from build123d import *

# Parameters (mm, degrees)
SKETCH1_W           = 125
SKETCH1_H           = 100
BOSS_EXTRUDE1_DEPTH = 15
SKETCH2_R           = 50
SKETCH2_R_2         = 37.5
BOSS_EXTRUDE2_DEPTH = 25
SKETCH5_R           = 20
BOSS_EXTRUDE3_DEPTH = 25
SKETCH6_R           = 15
CUT_EXTRUDE2_DEPTH  = 15


with BuildPart() as part:
    # Sketch1 → Boss-Extrude1 (new body)
    with BuildSketch(Plane(origin=(0, 0, 0), x_dir=(1, 0, 0), z_dir=(0, 1, 0))):
        Rectangle(SKETCH1_W, SKETCH1_H)
    boss_extrude1 = extrude(amount=BOSS_EXTRUDE1_DEPTH)

    # Sketch2 → Boss-Extrude2 (add)
    with BuildSketch(Plane.XZ):
        Circle(SKETCH2_R)
        Circle(SKETCH2_R_2, mode=Mode.SUBTRACT)
    extrude(amount=BOSS_EXTRUDE2_DEPTH)

    # Sketch5 → Boss-Extrude3 (add)
    with BuildSketch(Plane(origin=(62.5, 0, 0), x_dir=(0, 0, -1), z_dir=(1, 0, 0))):
        with BuildLine():
            ThreePointArc((-50, 100), (0, 150), (50, 100))
            Line((50, 100), (50, 15))
            Line((50, 15), (-50, 15))
            Line((-50, 15), (-50, 100))
        make_face()
        with Locations((0, 100)):
            Circle(SKETCH5_R, mode=Mode.SUBTRACT)
    boss_extrude3 = extrude(amount=-BOSS_EXTRUDE3_DEPTH)

    # Mirror1: Boss-Extrude1, Boss-Extrude3 across plane
    add(boss_extrude1.mirror(Plane(origin=(0, 0, 0), x_dir=(0, 0, 1), z_dir=(1, 0, 0))))
    add(boss_extrude3.mirror(Plane(origin=(0, 0, 0), x_dir=(0, 0, 1), z_dir=(1, 0, 0))))

    # Sketch6 → Cut-Extrude2 (cut)
    with BuildSketch(Plane.XZ):
        Circle(SKETCH6_R)
    extrude(amount=-CUT_EXTRUDE2_DEPTH, mode=Mode.SUBTRACT)


solid = part.part
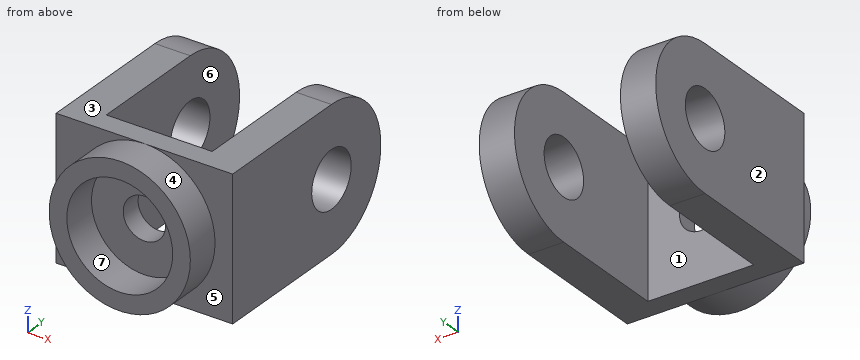
CAD build for the part. Positions are in the model's coordinates, mm. Face numbers are marked on the shaded views. A direction names the side the tool comes from. Round coordinates to 2 decimals unless told otherwise and drop trailing zeros. Loops run counter-clockwise (first coordinate to the right, second up) from the corner with the lowest first, then second, coordinate; pieces in that order, holes last. Notation, with made-up numbers: M -12,74 L 6,74 A31 ccw 6,105 Z; hole C 15,-19.75 d6. An arc over 180 degrees is marked long. One line per question, with ' | ' between items. Start each with the question number.
Item 1: Cut at C-C, the plane z = -18. Write the cut outline in (x, y), plus the area to 3 significant figures.
Item 2: Cut at A-A, the plane z = 0. Write the cut outline in (x, y), plus the area to 3 significant figures.
Item 3: Two-plate mould, pull along X, no slides. Class the marked faces 1, 2, 3 and 4: pulls with the +X half, pulls with the -X half, needs draft (parallel to the pull), parting line crosses it, or undercut.
Item 4: Cut at B-B, the plane y = 86.5. Write the cut outline in (x, z), plus the area to 3 significant figures.
Item 5: Cut at D-D, the plane y = -4. Write the cut outline in (x, z).
Item 6: Wall check: line 1 (X direction, y = 74, z = -30.5); line 2 (Y direction, x = 48.25, z = 0); line 3 (Y direction, x = 31, z = 25.5). Give the ranges that are in metal, low to high.
Item 7: Pin check, flat tips, straight feed: pin 1 Ø8 at (x, z) = (25, -15.5) entering from +Y; pin 2 Ø10 at (x, y) = (36.5, 75) entering from -Z. Stop position of each tip, or through.
Item 8: Which spindle directions (+Z, -Z, +X, -X, +Y, -Y) get a long thin tool onto all of the face, cutting with end or side? Do the marked faces 5, 6 and 7. Say none if no direction does.
Responses:
1) outline: M -62.5,0 L -46.65,0 L -46.65,-25 L -32.9,-25 L -32.9,0 L 32.9,0 L 32.9,-25 L 46.65,-25 L 46.65,0 L 62.5,0 L 62.5,91.28 L 37.5,91.28 L 37.5,15 L -37.5,15 L -37.5,91.28 L -62.5,91.28 Z; M -62.5,108.72 L -37.5,108.72 L -37.5,146.65 L -62.5,146.65 Z; M 37.5,108.72 L 62.5,108.72 L 62.5,146.65 L 37.5,146.65 Z | area: 8,270 mm²
2) outline: M -62.5,0 L -50,0 L -50,-25 L -37.5,-25 L -37.5,0 L -15,0 L -15,15 L -37.5,15 L -37.5,80 L -62.5,80 Z; M -62.5,120 L -37.5,120 L -37.5,150 L -62.5,150 Z; M 15,0 L 37.5,0 L 37.5,-25 L 50,-25 L 50,0 L 62.5,0 L 62.5,80 L 37.5,80 L 37.5,15 L 15,15 Z; M 37.5,120 L 62.5,120 L 62.5,150 L 37.5,150 Z | area: 6,800 mm²
3) face 1: undercut | face 2: pulls with the -X half | face 3: needs draft | face 4: parting line crosses it
4) outline: M -62.5,-50 L -37.5,-50 L -37.5,-14.76 L -62.5,-14.76 Z; M -62.5,14.76 L -37.5,14.76 L -37.5,50 L -62.5,50 Z; M 37.5,-50 L 62.5,-50 L 62.5,-14.76 L 37.5,-14.76 Z; M 37.5,14.76 L 62.5,14.76 L 62.5,50 L 37.5,50 Z | area: 3,520 mm²
5) outline: C 0,0 d100; hole C 0,0 d75
6) line 1: x = -62.5 to -37.5, 37.5 to 62.5 | line 2: y = -25 to 80, 120 to 150 | line 3: y = -25 to 15
7) pin 1: stops at y = 15 | pin 2: stops at z = -50
8) face 5: +X, -Y | face 6: +Z, -Z, +Y | face 7: -Y
